The figure shows three views and two pictorial views of one solid part (mm, origin at its lowest corner). Answer the questions. A direction names the side the tool comes from. Give positions to 0.01 mm unless a question says otherwise; leave off trailing zeros. Order: outer loops, then holes, each group sorted by start corner. A loop starts at its lowest first (then second) coordinate and runs counter-clockwise, first axis right, second up. Notation, with made-up numbers: M -29,17.25 L -21,17.25 A12 cw -21,28.25 Z; hole C 83,-25.75 d8. An arc over 180 degrees is marked long. One line per item, written item: value. Start each with the question number.
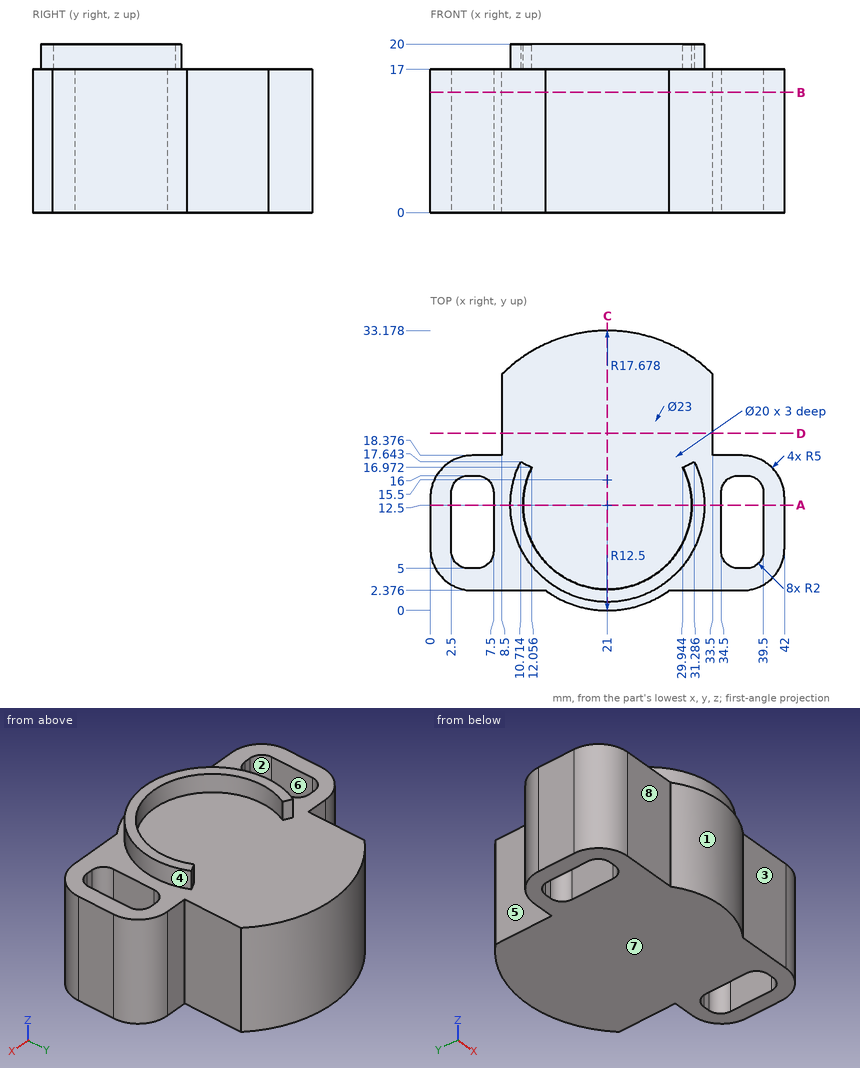
Q1. Consider probe 1 along X at (y, z) = (13.5, 10.75); probe 2 along X at (y, z) = (12.5, 19.3); probe 3 along Y at (x, z) = (21, 18.7). Determine where each line is inside the solid, lowest interval first.
Q2. Find section D-D, the plane y = 21. Give the vertices of the cut face in (x, z), then the cut area to 3 significant figures.
Q3. Find section A-A, the plane y = 12.5. Give the vertices of the cut face in (x, z).
Q4. A tool of negligible diameter and unlimited length cuts with its end or side. For the marked faces 4, 5, 6, 7 and 8, from which of +Z, -Z, +X, -X, +Y, -Y can it reach the whole face along a straight path? Write none if from no direction.
Q5. Each of these flat-tipped pins is pushed along its axis until it touches: pin 1 (12 mm diameter, centred on x = 17, y = 23.5, fed in from -Z); pin 2 (10 mm diameter, centred on y = 26, z = 14.5, fed in from -X); pin 3 (1 mm diameter, centred on y = 27.5, z = 3, fed in from +X); pin 4 (1.1 mm diameter, centred on x = 37, z = 6, fed in from -Y). Where does it stop, or does it pass through?
Q6. Find section B-B, the plane z = 14.25. State how many separate pieces and enclosed holes the cut face has, then the cut area to 3 significant figures.
Q7. Find section C-C, the plane x = 21. Give the vertices of the cut face in (y, z).
Q8. Determine the mould class of the marked faces 1, 2 and 3 for opening direction X: released by +X, released by -X, zero draft, split by the parting line, or undercut.
Evaluation:
1. probe 1: 0 to 2.5, 7.5 to 34.5, 39.5 to 42
1. probe 2: 9.5 to 11, 31 to 32.5
1. probe 3: 1 to 2.5
2. outline: M 8.5,0 L 33.5,0 L 33.5,17 L 8.5,17 Z
2. area: 425 mm2
3. outline: M 0,0 L 2.5,0 L 2.5,17 L 0,17 Z; M 7.5,0 L 34.5,0 L 34.5,17 L 32.5,17 L 32.5,20 L 31,20 L 31,17 L 11,17 L 11,20 L 9.5,20 L 9.5,17 L 7.5,17 Z; M 39.5,0 L 42,0 L 42,17 L 39.5,17 Z
4. face 4: +Z
4. face 5: +Z, -Z, -X, +Y
4. face 6: +Z, -Z
4. face 7: -Z, +X, -X, +Y, -Y
4. face 8: +Z, -Z, -X, -Y
5. pin 1: z = 0
5. pin 2: x = 8.5
5. pin 3: x = 33.5
5. pin 4: y = 2.38
6. separate pieces: 1
6. enclosed holes: 2
6. area: 901 mm2
7. outline: M 0,0 L 33.18,0 L 33.18,17 L 2.5,17 L 2.5,20 L 1,20 L 1,17 L 0,17 Z
8. face 1: split by the parting line
8. face 2: undercut
8. face 3: zero draft
